```python
from build123d import *

# Parameters (mm, degrees)
F0_W     = 2
F0_H     = 19
F0_W_2   = 28
F0_H_2   = 2
F0_W_3   = 24
F0_H_3   = 19.9385005981
F1_DEPTH = 65
F2_R     = 0.99999


# Not quite as in the source:
# - a fillet or chamfer is up to 0.001 mm smaller than in the source, because OpenCascade refuses the exact size


with BuildPart() as f1:
    # F0 (on Top) → F1 (new body)
    with BuildSketch(Plane.XY):
        with Locations((29, 32.5)):
            Rectangle(F0_W, F0_H)
        with Locations((14, 22)):
            Rectangle(F0_W_2, F0_H_2)
        with Locations((42, 22)):
            Rectangle(F0_W_3, F0_H_2)
        with Locations((55, 32.5)):
            Rectangle(F0_W, F0_H)
        with Locations((55, 22)):
            Rectangle(F0_W, F0_H_2)
        with Locations((68, 22)):
            Rectangle(F0_W_3, F0_H_2)
        with Locations((68, 1)):
            Rectangle(F0_W_3, F0_H_2)
        with Locations((55, 1)):
            Rectangle(F0_W, F0_H_2)
        with Locations((42, 1)):
            Rectangle(F0_W_3, F0_H_2)
        with Locations((14, 1)):
            Rectangle(F0_W_2, F0_H_2)
        with Locations((29, 1)):
            Rectangle(F0_W, F0_H_2)
        with Locations((29, 11.5)):
            Rectangle(F0_W, F0_H)
        with Locations((29, -9.5)):
            Rectangle(F0_W, F0_H)
        with Locations((55, -9.969250299)):
            Rectangle(F0_W, F0_H_3)
        with Locations((29, 22)):
            Rectangle(F0_W, F0_H_2)
        with Locations((55, 11.5)):
            Rectangle(F0_W, F0_H)
    extrude(amount=F1_DEPTH)

    # F2 (radius 1 in the source; OpenCascade refuses exactly that, so slightly less here)
    f2_edges = [f1.edges().sort_by_distance(p)[0] for p in [
        (28, 32.5, 65),
        (14, 23, 65),
        (0, 22, 65),
        (14, 21, 65),
        (28, 11.5, 65),
        (14, 2, 65),
        (0, 1, 65),
        (14, 0, 65),
        (28, -9.5, 65),
        (29, -19, 65),
        (30, -9.5, 65),
        (42, 0, 65),
        (54, -9.96925, 65),
        (55, -19.938501, 65),
        (56, -9.96925, 65),
        (68, 0, 65),
        (80, 1, 65),
        (68, 2, 65),
        (56, 11.5, 65),
        (68, 21, 65),
        (80, 22, 65),
        (68, 23, 65),
        (56, 32.5, 65),
        (55, 42, 65),
        (54, 32.5, 65),
        (42, 23, 65),
        (30, 32.5, 65),
        (29, 42, 65),
        (42, 2, 65),
        (30, 11.5, 65),
        (42, 21, 65),
        (54, 11.5, 65),
        (28, 32.5, 0),
        (14, 23, 0),
        (0, 22, 0),
        (14, 21, 0),
        (28, 11.5, 0),
        (14, 2, 0),
        (0, 1, 0),
        (14, 0, 0),
        (28, -9.5, 0),
        (29, -19, 0),
        (30, -9.5, 0),
        (42, 0, 0),
        (54, -9.96925, 0),
        (55, -19.938501, 0),
        (56, -9.96925, 0),
        (68, 0, 0),
        (80, 1, 0),
        (68, 2, 0),
        (56, 11.5, 0),
        (68, 21, 0),
        (80, 22, 0),
        (68, 23, 0),
        (56, 32.5, 0),
        (55, 42, 0),
        (54, 32.5, 0),
        (42, 23, 0),
        (30, 32.5, 0),
        (29, 42, 0),
        (42, 2, 0),
        (30, 11.5, 0),
        (42, 21, 0),
        (54, 11.5, 0),
        (30, 42, 32.5),
        (28, 42, 32.5),
        (56, 42, 32.5),
        (54, 42, 32.5),
        (0, 23, 32.5),
        (0, 21, 32.5),
        (0, 2, 32.5),
        (0, 0, 32.5),
        (28, -19, 32.5),
        (30, -19, 32.5),
        (54, -19.938501, 32.5),
        (56, -19.938501, 32.5),
        (80, 0, 32.5),
        (80, 2, 32.5),
        (80, 21, 32.5),
        (80, 23, 32.5),
    ]]
    fillet(f2_edges, radius=F2_R)


solid = f1.part
```
Can you work these out from the model? Positions are in its coordinate system, mm. A direction names the side the tool comes from. Coordinates: 2 decimals unless noted, no trailing zeros.
1) Which directions (+Z, -Z, +X, -X, +Y, -Y) give clear straight access to the entire face, cutting with the end or side of a thin tool? Please do faces 1 (the flat face through (68, 2, 32)), 2 (the flat face through (14, 21, 32)), 3 (the flat face through (42, 21, 32)), 4 (the flat face through (56, -10, 32)), 5 (the flat face through (54, 32, 32)).
2) I need wall thicknesses on probe 1 along X at (y, z) = (30, 30); probe 2 along Y at (x, z) = (20.5, 17.5); probe 3 along X at (y, z) = (21.5, 44.5). Which ranges of each line are inside material? Lowest first, please.
3) Thinking about a two-plate mould opening in Y: for faces 6 (the flat face through (14, 23, 32)), 7 (the flat face through (28, -9, 32)), 8 (the flat face through (56, 11, 32)), which applies, pulls with the +Y half, pulls with the -Y half, needs draft (parallel to the pull), parting line crosses it, or undercut?
4) For pin 1 (4 mm diameter, centred on x = 49.5, z = 34, fed in from +Y); pin 2 (2 mm diameter, centred on x = 9, z = 57.5, fed in from -Y); pin 3 (10 mm diameter, centred on x = 49.5, z = 10, fed in from -Y), each with a flat end and sliding along its axis, tell me the tip position at first contact or that it passes through.
Completed:
1. face 1: +Z, -Z, +X
1. face 2: +Z, -Z, -X
1. face 3: +Z, -Z
1. face 4: +Z, -Z, +X, -Y
1. face 5: +Z, -Z, +Y
2. probe 1: x = 28 to 30, 54 to 56
2. probe 2: y = 0 to 2, 21 to 23
2. probe 3: x = 0.13 to 79.87
3. face 6: pulls with the +Y half
3. face 7: needs draft
3. face 8: undercut
4. pin 1: stops at y = 23
4. pin 2: stops at y = 0
4. pin 3: stops at y = -19.8
